For this review, use the dimensioned drawing (mm, ordinates from the lowest corner) and the shaded views. A direction names the side the tool comes from. Round coordinates to 2 decimals unless told otherwise and drop trailing zeros. Write each loop counter-clockwise with the first axis right and the second up, starting at its lowest first coordinate (ties: lowest second). Pieces come first, ordered by that corner, then holes. Notation, with made-up numbers: (67.5, -35.75) -> (85.5, -35.75) arc R3 ccw to (85.5, -30.75) -> close; hole circle Ø5 at (55, 35). An arc over 180 degrees is marked (long way). Answer as CSV lines item,"result". Start each with the question number.
Item 1: Take a section at D-D on y = 59. Give the boundary of the cut face in (x, z) (1 decimal).
Item 2: Wall thickness on probe 1 along X at (y, z) = (17, 5.5) (1 decimal); probe 2 along X at (y, z) = (23, 14.5) (1 decimal); probe 3 along Y at (x, z) = (128, 20.25): over which ranges is each line inside the solid? List them lowest first. Write a range as from..to.
Item 3: Mouldability with a two-part tool opening along X and no side actions: class the marked faces 1, 2, 3 and 4 as +X half, -X half, draft (parallel to the pull), parting line (faces both ways), or undercut.
Item 4: Machinability: for the marked faces 5, 6 and 7, which of the approach directions +Z, -Z, +X, -X, +Y, -Y give a long, thin tool a straight path to every point of the face, cutting with its end or side? Answer none if there is none.
Item 5: For pin 1 Ø6.5 at (x, z) = (30, 10) entering from -Y; pin 2 Ø6 at (x, z) = (169, 10.5) entering from -Y (1 decimal); pin 3 Ø8 at (x, y) = (131.5, 23) entering from +Z; pin 4 Ø4.5 at (y, z) = (20.5, 8.5) entering from +X, all flat-tipped, find the tip position at first contact; note any pin that passes through.
Item 6: Take a section at B-B on z = 9.25. Give the boundary of the cut face in (x, y), then the cut area to 3 significant figures.
Item 7: Take a section at C-C on x = 78.5. Give the boundary of the cut face in (y, z), then the cut area to 3 significant figures.
Item 8: Take a section at A-A on y = 9.5. Give the boundary of the cut face in (x, z).
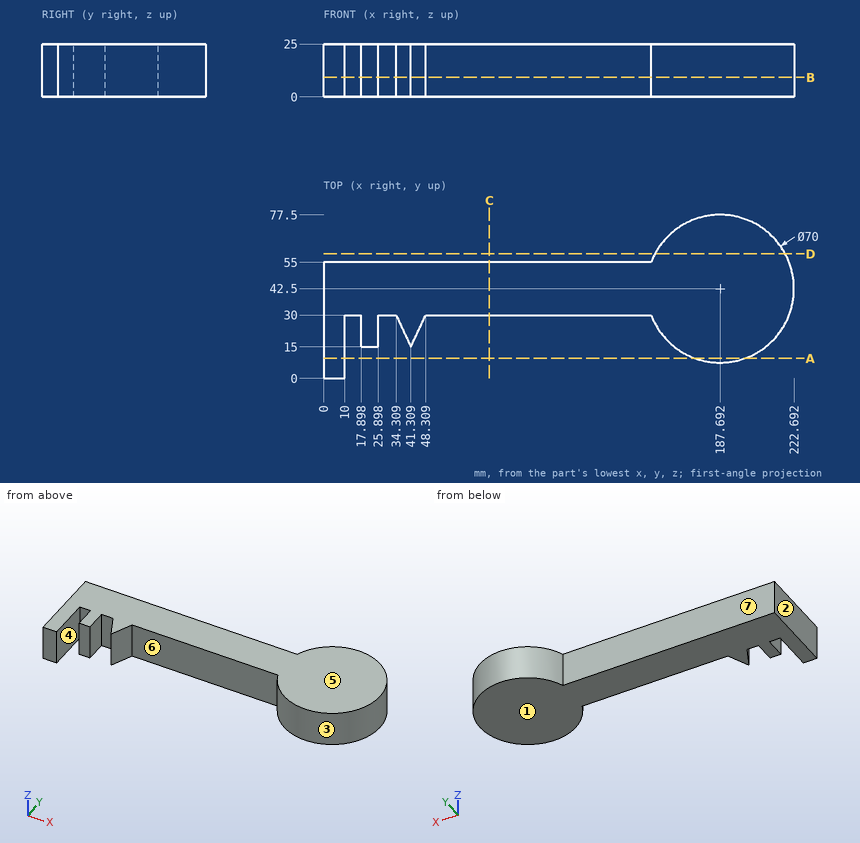
Output values:
1,outline,"(156.8, 0) -> (218.6, 0) -> (218.6, 25) -> (156.8, 25) -> close"
2,probe 1,"x = 0..10, 17.9..25.9, 40.4..42.2, 163.7..211.7"
2,probe 2,"x = 0..10, 17.9..25.9, 37.6..45, 158.6..216.8"
2,probe 3,"y = 30..55"
3,face 1,"draft"
3,face 2,"-X half"
3,face 3,"undercut"
3,face 4,"undercut"
4,face 5,"+Z, +X, -X, +Y, -Y"
4,face 6,"+Z, -Z, -Y"
4,face 7,"+Z, -Z, -X, +Y"
5,pin 1,"stops at y = 30"
5,pin 2,"stops at y = 11.2"
5,pin 3,"passes through"
5,pin 4,"stops at x = 216.59"
6,outline,"(0, 0) -> (10, 0) -> (10, 30) -> (17.9, 30) -> (17.9, 15) -> (25.9, 15) -> (25.9, 30) -> (34.31, 30) -> (41.31, 15) -> (48.31, 30) -> (155, 30) arc R35 ccw (long way) to (155, 55) -> (0, 55) -> close"
6,area,"8,210 mm^2"
7,outline,"(30, 0) -> (55, 0) -> (55, 25) -> (30, 25) -> close"
7,area,"625 mm^2"
8,outline,"(0, 0) -> (10, 0) -> (10, 25) -> (0, 25) -> close; (176.03, 0) -> (199.35, 0) -> (199.35, 25) -> (176.03, 25) -> close"
